```python
from build123d import *
from build123d.topology import SkipClean

# Parameters (mm, degrees)
SKETCH1_R           = 4
BOSS_EXTRUDE1_DEPTH = 7.5
CUT_EXTRUDE2_DEPTH  = 10
BOSS_EXTRUDE3_START = 8
SKETCH4_R           = 8.5
BOSS_EXTRUDE3_DEPTH = 8


with BuildPart() as part:
    # Sketch1 → Boss-Extrude1 (new body)
    with BuildSketch(Plane(origin=(0, 0, 0), x_dir=(1, 0, 0), z_dir=(0, 1, 0))):
        with Locations(Location((0, 0, 0), (0, 0, 270))):
            Circle(SKETCH1_R)
    extrude(amount=BOSS_EXTRUDE1_DEPTH)

    # Sketch2 → Cut-Extrude2 (cut)
    with BuildSketch(Plane(origin=(0, 0, 0), x_dir=(-1, 0, 0), z_dir=(0, -1, 0))):
        with BuildLine():
            Line((-2.190319611, -1.15), (2.190319611, -1.15))
            ThreePointArc((2.190319611, -1.15), (2.790247196, -0.202052895), (3, 0.9))
            ThreePointArc((3, 0.9), (-1.102052895, 3.690247196), (-2.190319611, -1.15))
        make_face()
    extrude(amount=-CUT_EXTRUDE2_DEPTH, mode=Mode.SUBTRACT)

    # Sketch4 → Boss-Extrude3 (add)
    with SkipClean():  # the faces are left unmerged after this step: merging them gives an invalid solid
        with BuildSketch(Plane(origin=(0, 0, 0), x_dir=(-1, 0, 0), z_dir=(0, -1, 0)).offset(BOSS_EXTRUDE3_START)):
            with Locations(Location((0, 0.9, 0), (0, 0, 90))):
                Circle(SKETCH4_R)
            with BuildLine():
                Line((2.190319611, -1.15), (-2.190319611, -1.15))
                ThreePointArc((-2.190319611, -1.15), (0, 3.9), (2.190319611, -1.15))
            make_face(mode=Mode.SUBTRACT)
        extrude(amount=-BOSS_EXTRUDE3_DEPTH)


solid = part.part
```
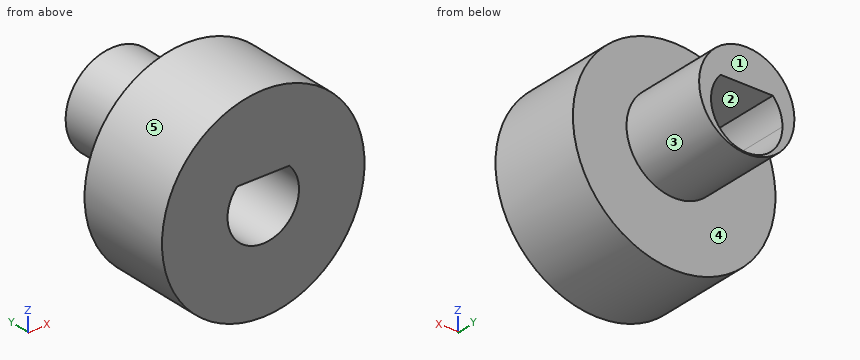
Work out the finished part from the listing and answer in its coordinate system (mm). Face numbers are marked on the shaded views. A direction names the side the tool comes from. Round coordinates to 2 decimals unless told otherwise and drop trailing zeros. Order: outer loops, then holes, each group sorted by start corner. A loop starts at its lowest first (then second) coordinate and runs counter-clockwise, first axis right, second up.
Q1. A tool of negligible diameter and unlimited length cuts with its end or side. For the marked faces 4 and 5, from which of +Z, -Z, +X, -X, +Y, -Y can it reach the whole face along a straight path? Write none if from no direction.
Solution:
face 4: +Y
face 5: +Y, -Y
Q2. A cutting plane is placed at A-A, the plane x = 0. Determine the outline of the cut face in (y, z), then the cut area to 3 significant figures.
Solution:
outline: (-8, -9.4) - (0, -9.4) - (0, -4) - (7.5, -4) - (7.5, -3.9) - (-8, -3.9) - close; (-8, 1.15) - (7.5, 1.15) - (7.5, 4) - (0, 4) - (0, 7.6) - (-8, 7.6) - close
area: 118 mm2
Q3. Given pin 1 Ø3 at (y, z) = (-4, -6) entering from -X; pin 2 Ø1 at (y, z) = (2.5, -2) entering from +X; pin 3 Ø5 at (x, z) = (0, -0.9) entering from +Y; pin 4 Ø6 at (x, y) = (-4, -5.5) entering from -Z, each flat-ended and moving along its own axis, determine where each tip first touches the part or whether it passes through.
Solution:
pin 1: stops at x = -7.7
pin 2: stops at x = 3.71
pin 3: stops at y = 7.5
pin 4: stops at z = -9.34
Q4. A cutting plane is placed at B-B, the plane z = 0. Determine the outline of the cut face in (x, y).
Solution:
outline: (-8.45, -8) - (-2.86, -8) - (-2.86, 7.5) - (-4, 7.5) - (-4, 0) - (-8.45, 0) - close; (2.86, -8) - (8.45, -8) - (8.45, 0) - (4, 0) - (4, 7.5) - (2.86, 7.5) - close
Q5. Find the intervals of material crossed by line 1 along X through (y, z) = (-4, -0.9); line 2 along Y through (x, z) = (-4, 3); line 3 along X through (y, z) = (2.25, -0.9), in increasing order.
Solution:
line 1: x = -8.5 to -3, 3 to 8.5
line 2: y = -8 to 0
line 3: x = -3.9 to -3, 3 to 3.9
Q6. A cutting plane is placed at D-D, the plane z = -2. Determine the outline of the cut face in (x, y).
Solution:
outline: (-8.43, -8) - (-2.79, -8) - (-2.79, 7.5) - (-3.46, 7.5) - (-3.46, 0) - (-8.43, 0) - close; (2.79, -8) - (8.43, -8) - (8.43, 0) - (3.46, 0) - (3.46, 7.5) - (2.79, 7.5) - close
Q7. A cutting plane is placed at C-C, the plane y = 3.25. Determine the outline of the cut face in (x, z), then the cut area to 3 significant figures.
Solution:
outline: circle Ø8 at (0, 0); hole (-2.19, 1.15) arc R3 ccw (long way) to (2.19, 1.15) - close
area: 24.9 mm2
Q8. The mould has two halves that part along X. Classify the marked faces 1, 2 and 3: pulls with the +X half, pulls with the -X half, needs draft (parallel to the pull), parting line crosses it, or undercut.
Solution:
face 1: needs draft
face 2: undercut
face 3: parting line crosses it
